from build123d import *

# Parameters (mm, degrees)
SKETCH006_W       = 19
SKETCH006_H       = 19
PAD004_DEPTH      = 5
PAD004_DEPTH_BACK = 14
CHAMFER001_SIZE   = 3
PAD005_DEPTH      = 36.7


with BuildPart() as part:
    # Sketch006 → Pad004 (new body, two sides)
    with BuildSketch(Plane.XY) as pad004_sk:
        Rectangle(SKETCH006_W, SKETCH006_H)
    extrude(amount=PAD004_DEPTH)
    extrude(pad004_sk.sketch, amount=-PAD004_DEPTH_BACK)

    # Chamfer001
    chamfer001_edges = [part.edges().sort_by_distance(p)[0] for p in [
        (9.5, 9.5, -4.5),
        (-9.5, 9.5, -4.5),
        (0, 9.5, -14),
        (-9.5, 0, -14),
        (9.5, 0, -14),
        (-9.5, 0, 5),
        (9.5, 0, 5),
    ]]
    chamfer(chamfer001_edges, length=CHAMFER001_SIZE)

    # Chamfer001 Face8 → Pad005 (add)
    with BuildSketch(Plane(origin=(0, -9.5, -4.5), x_dir=(-1, 0, 0), z_dir=(0, -1, 0))):
        Polygon((-9.5, 6.5), (-9.5, -6.5), (-6.5, -9.5), (6.5, -9.5), (9.5, -6.5), (9.5, 6.5), (6.5, 9.5), (-6.5, 9.5), align=None)
    extrude(amount=PAD005_DEPTH)


solid = part.part
Can you work these out from the model? Positions are in its coordinate system, mm. Give positions to 0.01 mm unless a question says otherwise; leave off trailing zeros. Loops run counter-clockwise (first coordinate to the right, second up) from the corner with the lowest first, then second, coordinate; pieces in that order, holes last. Notation, with made-up numbers: (-31, 16) -> (-24, 16) arc R14 ccw to (-24, 35) -> close; hole circle Ø2 at (70, -5). An arc over 180 degrees is marked (long way). Use one line per item in the form item = value.
1) If we section it at C-C (x = 8.25): Please give me the cut outline in (y, z).
Answers:
outline = (-46.2, -12.25) -> (6.5, -12.25) -> (7.75, -11) -> (7.75, 3.25) -> (-46.2, 3.25) -> close
2) If we section it at B-B (y = -10): Please give me the cut outline in (x, z), plus the area to 3 significant figures.
Answers:
outline = (-9.5, -11) -> (-6.5, -14) -> (6.5, -14) -> (9.5, -11) -> (9.5, 2) -> (6.5, 5) -> (-6.5, 5) -> (-9.5, 2) -> close
area = 343 mm²
3) If we section it at A-A (z = 3.5): Please give me the cut outline in (x, y), plus the area to 3 significant figures.
Answers:
outline = (-8, -46.2) -> (8, -46.2) -> (8, 8) -> (6.5, 9.5) -> (-6.5, 9.5) -> (-8, 8) -> close
area = 889 mm²
4) I need wall thicknesses on line 1 along Y through (x, z) = (-2.5, -11.25); line 2 along Z through (x, y) = (-7.25, 2); line 3 along Z through (x, y) = (8, 6). Which ranges of each line are inside material? Lowest first, please.
Answers:
line_1 = -46.2 to 9.25
line_2 = -13.25 to 4.25
line_3 = -12.5 to 3.5
5) If we section it at D-D (z = -12): Please give me the cut outline in (x, y).
Answers:
outline = (-8.5, -46.2) -> (8.5, -46.2) -> (8.5, 6.5) -> (6.5, 8.5) -> (-6.5, 8.5) -> (-8.5, 6.5) -> close
